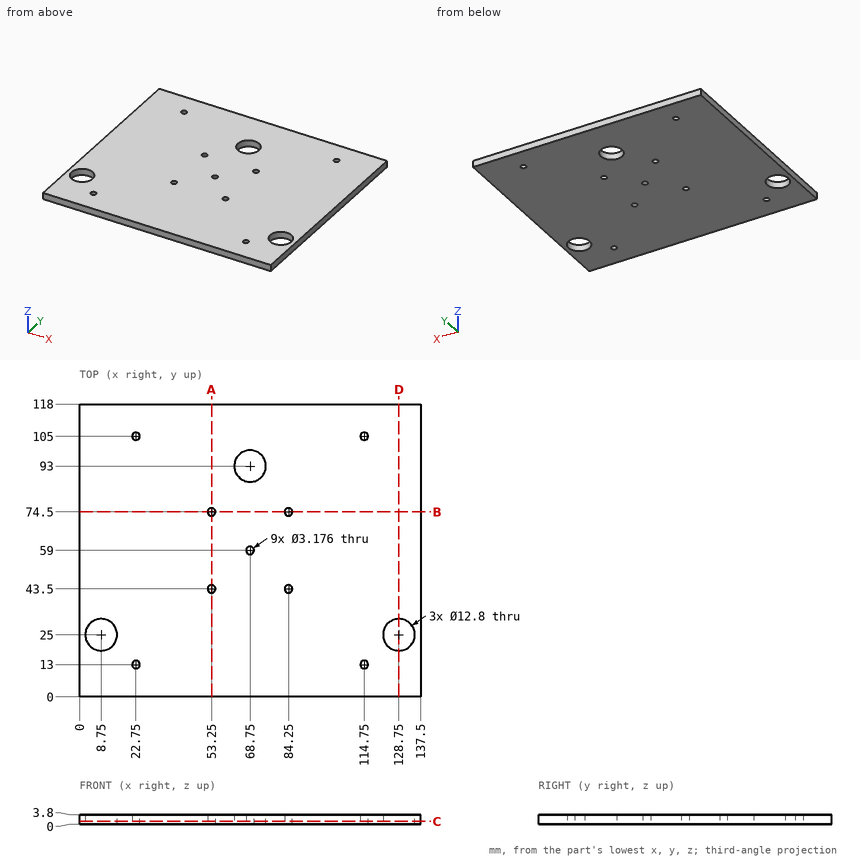
The figure shows three views and two pictorial views of one solid part (mm, origin at its lowest corner). Answer the questions. Coordinates: 2 decimals unless noted, no trailing zeros. Loops run counter-clockwise (first coordinate to the right, second up) from the corner with the lowest first, then second, coordinate; pieces in that order, holes last. Notation, with made-up numbers: (84, -5) - (143, -5) arc R10 cw to (143, 5) - close; hole circle Ø11 at (59.25, 30.25). An arc over 180 degrees is marked (long way). Use a Markdown table: item, result. Add a question column.
1) The part is cut by section A-A, the plane x = 53.25. Give the vertices of the cut face in (y, z), and give its area (3 significant figures).
2) The part is cut by section C-C, the plane z = 1.2. State how many separate pieces and enclosed holes the cut face has, and give its area (3 significant figures).
3) Find the intervals of material crossed by line 1 (Y direction, x = 68.75, z = 2.5); line 2 (Y direction, x = 84.25, z = 1.05); line 3 (X direction, y = 74.5, z = 0.8), in increasing order.
4) The part is cut by section D-D, the plane x = 128.75. Give the vertices of the cut face in (y, z).
5) The part is cut by section B-B, the plane y = 74.5. Give the vertices of the cut face in (x, z), and give its area (3 significant figures).
Here are the results:
| question | item | result |
|---|---|---|
| 1 | outline | (0, 0) - (41.91, 0) - (41.91, 3.8) - (0, 3.8) - close; (45.09, 0) - (72.91, 0) - (72.91, 3.8) - (45.09, 3.8) - close; (76.09, 0) - (118, 0) - (118, 3.8) - (76.09, 3.8) - close |
| 1 | area | 424 mm^2 |
| 2 | separate pieces | 1 |
| 2 | enclosed holes | 12 |
| 2 | area | 15,800 mm^2 |
| 3 | line 1 | y = 0 to 57.41, 60.59 to 86.6, 99.4 to 118 |
| 3 | line 2 | y = 0 to 41.91, 45.09 to 72.91, 76.09 to 118 |
| 3 | line 3 | x = 0 to 51.66, 54.84 to 82.66, 85.84 to 137.5 |
| 4 | outline | (0, 0) - (18.6, 0) - (18.6, 3.8) - (0, 3.8) - close; (31.4, 0) - (118, 0) - (118, 3.8) - (31.4, 3.8) - close |
| 5 | outline | (0, 0) - (51.66, 0) - (51.66, 3.8) - (0, 3.8) - close; (54.84, 0) - (82.66, 0) - (82.66, 3.8) - (54.84, 3.8) - close; (85.84, 0) - (137.5, 0) - (137.5, 3.8) - (85.84, 3.8) - close |
| 5 | area | 498 mm^2 |
